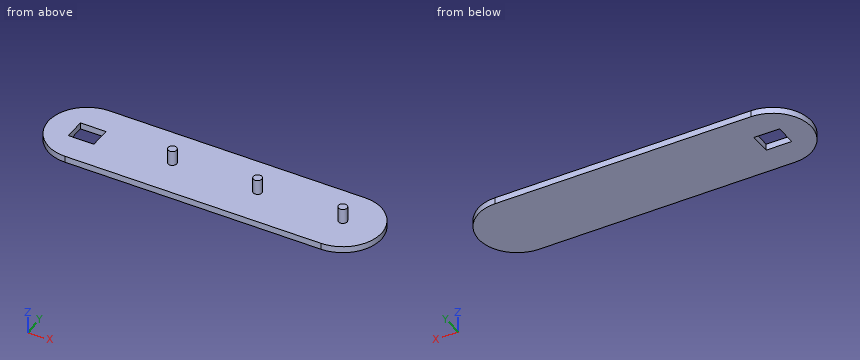
```python
from build123d import *

# Parameters (mm, degrees)
BOSS_EXTRUDE1_DEPTH = 3
SKETCH3_W           = 12
SKETCH3_H           = 10
CUT_EXTRUDE1_DEPTH  = 3
SKETCH5_R           = 2
BOSS_EXTRUDE2_DEPTH = 7
LPATTERN1_COUNT     = 4
LPATTERN1_PITCH     = 40


with BuildPart() as part:
    # Sketch2 → Boss-Extrude1 (new body)
    with BuildSketch(Plane.XY):
        with BuildLine():
            Line((0, 18), (120, 18))
            ThreePointArc((120, 18), (138, 0), (120, -18))
            Line((120, -18), (0, -18))
            ThreePointArc((0, -18), (-18, 0), (0, 18))
        make_face()
    extrude(amount=BOSS_EXTRUDE1_DEPTH)

    # Sketch3 → Cut-Extrude1 (cut)
    with BuildSketch(Plane.XY.offset(3)):
        Rectangle(SKETCH3_W, SKETCH3_H)
    extrude(amount=-CUT_EXTRUDE1_DEPTH, mode=Mode.SUBTRACT)

    # Sketch5 → Boss-Extrude2 (add)
    with BuildSketch(Plane.XY.offset(3)):
        with Locations((120, 0)):
            Circle(SKETCH5_R)
    boss_extrude2 = extrude(amount=BOSS_EXTRUDE2_DEPTH)

    # LPattern1: Boss-Extrude2 ×4, 1 skipped
    with Locations(*[(-i * LPATTERN1_PITCH, 0, 0) for i in range(1, LPATTERN1_COUNT) if i not in (3,)]):
        add(boss_extrude2)


solid = part.part
```
Check sheet for the modelled part. Datum: model origin and axes. Units: mm. Round coordinates to 2 decimals unless told otherwise and drop trailing zeros. Order: outer loops, then holes, each group sorted by start corner. A loop starts at its lowest first (then second) coordinate and runs counter-clockwise, first axis right, second up.
1) Go/stop test with flat-tipped pins: pin 1 Ø2 at (x, y) = (63.5, -6) entering from -Z; pin 2 Ø12 at (x, y) = (48.5, 0) entering from +Z; pin 3 Ø6 at (y, z) = (4, 5) entering from +X; pin 4 Ø2 at (y, z) = (2, 4.5) entering from +X. Record where each tip stops, or that it passes through.
2) Section check B-B (x = 80). Record the boundary of the cut face in (y, z).
3) Section check A-A (y = 0). Record the boundary of the cut face in (x, z), and give its area (3 significant figures).
4) Section check C-C (z = 6.25). Record the boundary of the cut face in (x, y), and give its area (3 significant figures).
5) Scan lines: line 1 (Z direction, x = 108, y = -9.5); line 2 (Y direction, x = 2, z = 1.5); line 3 (Y direction, x = 129, z = 1). Record each from-to range of solid material in increasing order.
6) Section check D-D (y = 16.5). Record the boundary of the cut face in (x, z).
Result:
1. pin 1: stops at z = 0
1. pin 2: stops at z = 3
1. pin 3: stops at x = 137.91
1. pin 4: stops at x = 121.73
2. outline: (-18, 0) - (18, 0) - (18, 3) - (2, 3) - (2, 10) - (-2, 10) - (-2, 3) - (-18, 3) - close
3. outline: (-18, 0) - (-6, 0) - (-6, 3) - (-18, 3) - close; (6, 0) - (138, 0) - (138, 3) - (122, 3) - (122, 10) - (118, 10) - (118, 3) - (82, 3) - (82, 10) - (78, 10) - (78, 3) - (42, 3) - (42, 10) - (38, 10) - (38, 3) - (6, 3) - close
3. area: 516 mm2
4. outline: circle Ø4 at (40, 0); circle Ø4 at (80, 0); circle Ø4 at (120, 0)
4. area: 37.7 mm2
5. line 1: z = 0 to 3
5. line 2: y = -18 to -5, 5 to 18
5. line 3: y = -15.59 to 15.59
6. outline: (-7.19, 0) - (127.19, 0) - (127.19, 3) - (-7.19, 3) - close
